Can you work these out from the model? Positions are in its coordinate system, mm. Round coordinates to 2 decimals unless told otherwise and drop trailing zeros. Loops run counter-clockwise (first coordinate to the right, second up) from the corner with the lowest first, then second, coordinate; pieces in that order, holes last. Notation, with made-up numbers: M 12.5,65 L 30.5,65 A19 ccw 30.5,78 Z; hole C 42.5,-14.5 d5. An arc over 180 degrees is marked long. Use a Markdown table: item, result. Add a question column.
```python
from build123d import *

# Parameters (mm, degrees)
SKETCH1_W           = 205.74
SKETCH1_H           = 133.35
BOSS_EXTRUDE1_DEPTH = 3.175
SKETCH3_R           = 3.175
CUT_EXTRUDE3_DEPTH  = 123.629006153
SKETCH4_R           = 3.175
CUT_EXTRUDE4_DEPTH  = 123.629006153
CUT_EXTRUDE5_DEPTH  = 123.629006153


with BuildPart() as part:
    # Sketch1 → Boss-Extrude1 (new body)
    with BuildSketch(Plane(origin=(0, 0, 0), x_dir=(1, 0, 0), z_dir=(0, 1, 0))):
        Rectangle(SKETCH1_W, SKETCH1_H)
    extrude(amount=BOSS_EXTRUDE1_DEPTH)

    # Sketch3 → Cut-Extrude3 (cut, through all)
    with BuildSketch(Plane(origin=(0, 3.175, 0), x_dir=(1, 0, 0), z_dir=(0, 1, 0))):
        with Locations(Location((35.56, 33.812500066, 0), (0, 0, 270))):
            Circle(SKETCH3_R)
        with Locations(Location((35.56, -33.812500066, 0), (0, 0, 270))):
            Circle(SKETCH3_R)
        with Locations(Location((-33.02, -33.812500066, 0), (0, 0, 270))):
            Circle(SKETCH3_R)
        with Locations(Location((-33.02, 33.812500066, 0), (0, 0, 270))):
            Circle(SKETCH3_R)
    extrude(amount=-CUT_EXTRUDE3_DEPTH, mode=Mode.SUBTRACT)

    # Sketch4 → Cut-Extrude4 (cut, through all)
    with BuildSketch(Plane(origin=(0, 3.175, 0), x_dir=(1, 0, 0), z_dir=(0, 1, 0))):
        with Locations(Location((-93.345, 57.15, 0), (0, 0, 270))):
            Circle(SKETCH4_R)
        with Locations(Location((93.345, 57.15, 0), (0, 0, 270))):
            Circle(SKETCH4_R)
        with Locations(Location((93.345, -57.15, 0), (0, 0, 90))):
            Circle(SKETCH4_R)
        with Locations(Location((-93.345, -57.15, 0), (0, 0, 90))):
            Circle(SKETCH4_R)
    extrude(amount=-CUT_EXTRUDE4_DEPTH, mode=Mode.SUBTRACT)

    # Sketch5 → Cut-Extrude5 (cut, through all)
    with BuildSketch(Plane(origin=(0, 3.175, 0), x_dir=(1, 0, 0), z_dir=(0, 1, 0))):
        with BuildLine():
            Line((-54.61, -42.545), (54.61, -42.545))
            ThreePointArc((54.61, -42.545), (56.406051224, -43.288948776), (57.15, -45.085))
            Line((57.15, -45.085), (57.15, -46.355))
            ThreePointArc((57.15, -46.355), (56.406051224, -48.151051224), (54.61, -48.895))
            Line((54.61, -48.895), (-54.61, -48.895))
            ThreePointArc((-54.61, -48.895), (-56.406051224, -48.151051224), (-57.15, -46.355))
            Line((-57.15, -46.355), (-57.15, -45.085))
            ThreePointArc((-57.15, -45.085), (-56.406051224, -43.288948776), (-54.61, -42.545))
        make_face()
        with BuildLine():
            Line((57.15, 45.085), (57.15, 46.355))
            ThreePointArc((57.15, 46.355), (56.406051224, 48.151051224), (54.61, 48.895))
            Line((54.61, 48.895), (-54.61, 48.895))
            ThreePointArc((-54.61, 48.895), (-56.406051224, 48.151051224), (-57.15, 46.355))
            Line((-57.15, 46.355), (-57.15, 45.085))
            ThreePointArc((-57.15, 45.085), (-56.406051224, 43.288948776), (-54.61, 42.545))
            Line((-54.61, 42.545), (54.61, 42.545))
            ThreePointArc((54.61, 42.545), (56.406051224, 43.288948776), (57.15, 45.085))
        make_face()
    extrude(amount=-CUT_EXTRUDE5_DEPTH, mode=Mode.SUBTRACT)


solid = part.part
```
(1) Suppose I cut it at D-D on y = 0.65. Count the separate pieces of the cut face and the enclosed holes in it, and give its area (3 significant figures).
(2) Suppose I cut it at A-A on x = 35.56. List the corners of the cut face in (y, z) for me (1 decimal), and give its area (3 significant figures).
(3) Suppose I cut it at C-C on x = 14. List the corners of the cut face in (y, z) for me (3 decimals).
(4) Suppose I cut it at B-B on z = 57.15. List the corners of the cut face in (x, y) for me (3 decimals).
(5) If I drill on probe 1 along Z at (x, y) = (-25, 2.25) (3 decimals); probe 2 along X at (y, z) = (1.4, -57.15); probe 3 along X at (y, z) = (2.25, 33.5), over which ranges is the centre line in solid material (lowest first)? Write a range as [from, to].
(6) Thinking about a two-plate mould opening in Z: for faces 1 (the face through (-1, 3.175, -1)), 2 (the face through (-34.24, 1.61, -30.88)), which applies, released by +Z, released by -Z, zero draft, split by the parting line, or undercut?
Results below:
| question | item | result |
|---|---|---|
| 1 | separate pieces | 1 |
| 1 | enclosed holes | 10 |
| 1 | area | 25,700 mm² |
| 2 | outline | M 0,-66.7 L 3.2,-66.7 L 3.2,-48.9 L 0,-48.9 Z; M 0,-42.5 L 3.2,-42.5 L 3.2,-37 L 0,-37 Z; M 0,-30.6 L 3.2,-30.6 L 3.2,30.6 L 0,30.6 Z; M 0,37 L 3.2,37 L 3.2,42.5 L 0,42.5 Z; M 0,48.9 L 3.2,48.9 L 3.2,66.7 L 0,66.7 Z |
| 2 | area | 343 mm² |
| 3 | outline | M 0,-66.675 L 3.175,-66.675 L 3.175,-48.895 L 0,-48.895 Z; M 0,-42.545 L 3.175,-42.545 L 3.175,42.545 L 0,42.545 Z; M 0,48.895 L 3.175,48.895 L 3.175,66.675 L 0,66.675 Z |
| 4 | outline | M -102.87,0 L -96.52,0 L -96.52,3.175 L -102.87,3.175 Z; M -90.17,0 L 90.17,0 L 90.17,3.175 L -90.17,3.175 Z; M 96.52,0 L 102.87,0 L 102.87,3.175 L 96.52,3.175 Z |
| 5 | probe 1 | z = [-66.675, -48.895], [-42.545, 42.545], [48.895, 66.675] |
| 5 | probe 2 | x = [-102.87, -96.52], [-90.17, 90.17], [96.52, 102.87] |
| 5 | probe 3 | x = [-102.87, -36.18], [-29.86, 32.4], [38.72, 102.87] |
| 6 | face 1 | zero draft |
| 6 | face 2 | undercut |
